```python
from build123d import *

# Parameters (mm, degrees)
F0_W     = 60.5891123414
F0_H     = 39.380852133
F1_DEPTH = 590
F2_DEPTH = 260
F3_DEPTH = 262
F4_R     = 5
F5_T     = -1


with BuildPart() as f1:
    # F0 (on Top) → F1 (new body)
    with BuildSketch(Plane.XY):
        with Locations((30.2945561707, -19.6904260665)):
            Rectangle(F0_W, F0_H)
    extrude(amount=F1_DEPTH)

    # F2 (add): a face of the model
    f2_faces = [f1.faces().sort_by_distance(p)[0] for p in [
        (0, -19.6904260665, 295),
    ]]
    extrude(f2_faces, amount=-F2_DEPTH)

    # F3 (add): a face of the model
    f3_faces = [f1.faces().sort_by_distance(p)[0] for p in [
        (130, 0, 295),
    ]]
    extrude(f3_faces, amount=-F3_DEPTH)

    # F4
    f4_edges = [f1.edges().sort_by_distance(p)[0] for p in [
        (0, -262, 295),
        (260, -262, 295),
    ]]
    fillet(f4_edges, radius=F4_R)

    # F5
    f5_openings = [f1.faces().sort_by_distance(p)[0] for p in [
        (130, -130.979538, 590),
        (130, 0, 295),
        (130, -130.979538, 0),
    ]]
    offset(amount=F5_T, openings=f5_openings)


solid = f1.part
```
Here's how the part is built. I have some questions about the finished solid (model axes, mm). A direction names the side the tool comes from. Coordinates: 2 decimals unless noted, no trailing zeros. Order: outer loops, then holes, each group sorted by start corner. A loop starts at its lowest first (then second) coordinate and runs counter-clockwise, first axis right, second up. Notation, with made-up numbers: (-23, 4.5) - (14, 4.5) arc R10 cw to (14, 8.5) - close; hole circle Ø9 at (25, 85). An arc over 180 degrees is marked (long way). One line per question, with ' | ' between items.
(1) Suppose I cut it at A-A on y = -178. List the corners of the cut face in (x, z) for me, and give its area (3 significant figures).
Report:
outline: (0, 0) - (1, 0) - (1, 590) - (0, 590) - close; (259, 0) - (260, 0) - (260, 590) - (259, 590) - close | area: 1,180 mm2
(2) Suppose I cut it at C-C on x = 150. List the corners of the cut face in (y, z) for me, and give its area (3 significant figures).
Report:
outline: (-262, 0) - (-261, 0) - (-261, 590) - (-262, 590) - close | area: 590 mm2
(3) Will this pin go through, and if not, where does the flat tip stop? pin 1 (1 mm diameter, centred on x = 174, z = 404.5, fed in from +Y).
Report:
pin 1: stops at y = -261
(4) Suppose I cut it at B-B on z = 183.5. List the corners of the cut face in (x, y) for me, and give its area (3 significant figures).
Report:
outline: (0, -257) arc R5 ccw to (5, -262) - (255, -262) arc R5 ccw to (260, -257) - (260, 0) - (259, 0) - (259, -257) arc R4 cw to (255, -261) - (5, -261) arc R4 cw to (1, -257) - (1, 0) - (0, 0) - close | area: 778 mm2
(5) If I drill on L1, parallel to X at y = -240.5, z = 200.5; L2, parallel to Y at x = 137.5, z = 327.5, over which ranges is the centre line in solid material (lowest first)?
Report:
L1: x = 0 to 1, 259 to 260 | L2: y = -262 to -261
(6) If we mould it in two halves opening along X, with no side actions, what happens to faces 3 (the flat face through (260, -127, 291)), 4 (the flat face through (128, -261, 291)), 5 (the flat face through (0, -127, 291))? For each: pulls with the +X half, pulls with the -X half, needs draft (parallel to the pull), parting line crosses it, or undercut.
Report:
face 3: pulls with the +X half | face 4: undercut | face 5: pulls with the -X half
(7) For faces 1 (the flat face through (128, -262, 291)), 2 (the flat face through (1, -127, 291)), which set-ups out of +Z, -Z, +X, -X, +Y, -Y let a thin tool reach every point of the face, with its end or its side?
Report:
face 1: +Z, -Z, +X, -X, -Y | face 2: +Z, -Z, +Y
